The listing builds one solid part. Answer for the finished solid, in the listing's coordinates (mm). Round coordinates to 2 decimals unless told otherwise and drop trailing zeros. Loops run counter-clockwise (first coordinate to the right, second up) from the corner with the lowest first, then second, coordinate; pieces in that order, holes last. Notation, with made-up numbers: (44, 16) -> (87, 16) arc R21 ccw to (87, 29) -> close; hole circle Ø7 at (16, 81). An arc over 180 degrees is marked (long way). Write each question's results on one line, items separated by ' | '. Start each with the question number.
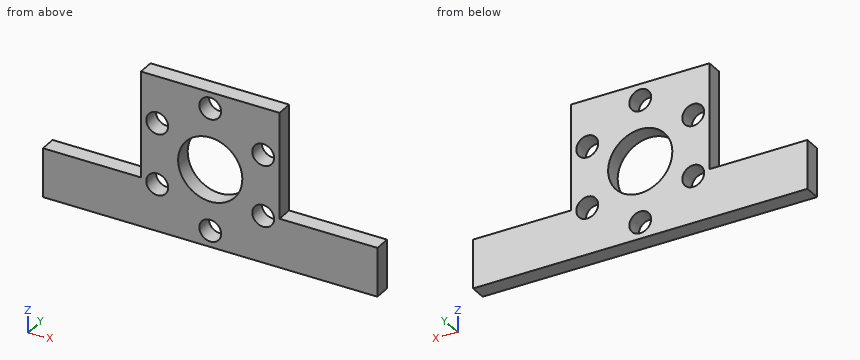
from build123d import *

# Parameters (mm, degrees)
SKETCH1_R            = 5
BOSS_EXTRUDE1_DEPTH  = 2.54
M3_CLEARANCE_HOLE1_D = 3.4


with BuildPart() as part:
    # Sketch1 → Boss-Extrude1 (new body)
    with BuildSketch(Plane(origin=(0, 0, 0), x_dir=(1, 0, 0), z_dir=(0, 1, 0))):
        Polygon((10.788891971, 4.445), (26.028891971, 4.445), (26.028891971, 12.065), (-26.028891971, 12.065), (-26.028891971, 4.445), (-10.788891971, 4.445), (-10.788891971, -12.065), (10.788891971, -12.065), align=None)
        with Locations(Location((0, 0, 0), (0, 0, 270))):
            Circle(SKETCH1_R, mode=Mode.SUBTRACT)
    extrude(amount=BOSS_EXTRUDE1_DEPTH)

    # M3 Clearance Hole1 (through all)
    with Locations(Plane(origin=(0, 2.54, 0), x_dir=(1, 0, 0), z_dir=(0, 1, 0))):
        with Locations((0, 9.525), (8.248891971, 4.7625), (8.248891971, -4.7625), (0, -9.525), (-8.248891971, -4.7625), (-8.248891971, 4.7625)):
            Hole(M3_CLEARANCE_HOLE1_D / 2)


solid = part.part
Item 1: Straight lines are drawn through the part: L1, parallel to X at y = 1.2, z = 6; L2, parallel to X at y = 0.95, z = 0; L3, parallel to X at y = 1, z = -3.75. For each, find the intervals that lie inside material, in ascending order. Write a range as [from, to].
Item 2: The part is cut by section B-B, the plane z = 0. Give the vertices of the cut face in (x, y).
Item 3: Each of these flat-tipped pins is pushed along its axis until it touches: pin 1 Ø1.5 at (y, z) = (0.5, 0.5) entering from -X; pin 2 Ø0.8 at (x, y) = (-22, 1) entering from +Z (3 decimals). Where does it stop, or does it pass through?
Item 4: The part is cut by section C-C, the plane x = -8.5. Give the vertices of the cut face in (y, z) (3 decimals), plus the area to 3 significant figures.
Item 5: The part is cut by section D-D, the plane y = 0.8. Give the vertices of the cut face in (x, z) (1 decimal), plus the area to 3 significant figures.
Item 6: The part is cut by section A-A, the plane x = 0. Give the vertices of the cut face in (y, z) (3 decimals), plus the area to 3 significant figures.
Report:
1) L1: x = [-10.79, -9.41], [-7.08, 7.08], [9.41, 10.79] | L2: x = [-10.79, -5], [5, 10.79] | L3: x = [-10.79, -9.61], [-6.88, -3.31], [3.31, 6.88], [9.61, 10.79]
2) outline: (-10.79, 0) -> (-5, 0) -> (-5, 2.54) -> (-10.79, 2.54) -> close; (5, 0) -> (10.79, 0) -> (10.79, 2.54) -> (5, 2.54) -> close
3) pin 1: stops at x = -10.79 | pin 2: stops at z = -4.445
4) outline: (0, -12.065) -> (2.54, -12.065) -> (2.54, -6.444) -> (0, -6.444) -> close; (0, -3.081) -> (2.54, -3.081) -> (2.54, 3.081) -> (0, 3.081) -> close; (0, 6.444) -> (2.54, 6.444) -> (2.54, 12.065) -> (0, 12.065) -> close | area: 44.2 mm2
5) outline: (-26, -12.1) -> (26, -12.1) -> (26, -4.4) -> (10.8, -4.4) -> (10.8, 12.1) -> (-10.8, 12.1) -> (-10.8, -4.4) -> (-26, -4.4) -> close; hole circle Ø3.4 at (-8.2, -4.8); hole circle Ø3.4 at (-8.2, 4.8); hole circle Ø10 at (0, 0); hole circle Ø3.4 at (0, -9.5); hole circle Ø3.4 at (0, 9.5); hole circle Ø3.4 at (8.2, -4.8); hole circle Ø3.4 at (8.2, 4.8) | area: 620 mm2
6) outline: (0, -12.065) -> (2.54, -12.065) -> (2.54, -11.225) -> (0, -11.225) -> close; (0, -7.825) -> (2.54, -7.825) -> (2.54, -5) -> (0, -5) -> close; (0, 5) -> (2.54, 5) -> (2.54, 7.825) -> (0, 7.825) -> close; (0, 11.225) -> (2.54, 11.225) -> (2.54, 12.065) -> (0, 12.065) -> close | area: 18.6 mm2
